Could you check a few things on this drawing? It's one solid part, dimensions in mm from its lowest x, y, z. A direction names the side the tool comes from. Give positions to 0.01 mm unless a question says otherwise; leave off trailing zeros. Order: outer loops, then holes, each group sorted by start corner. A loop starts at its lowest first (then second) coordinate and runs counter-clockwise, first axis right, second up.
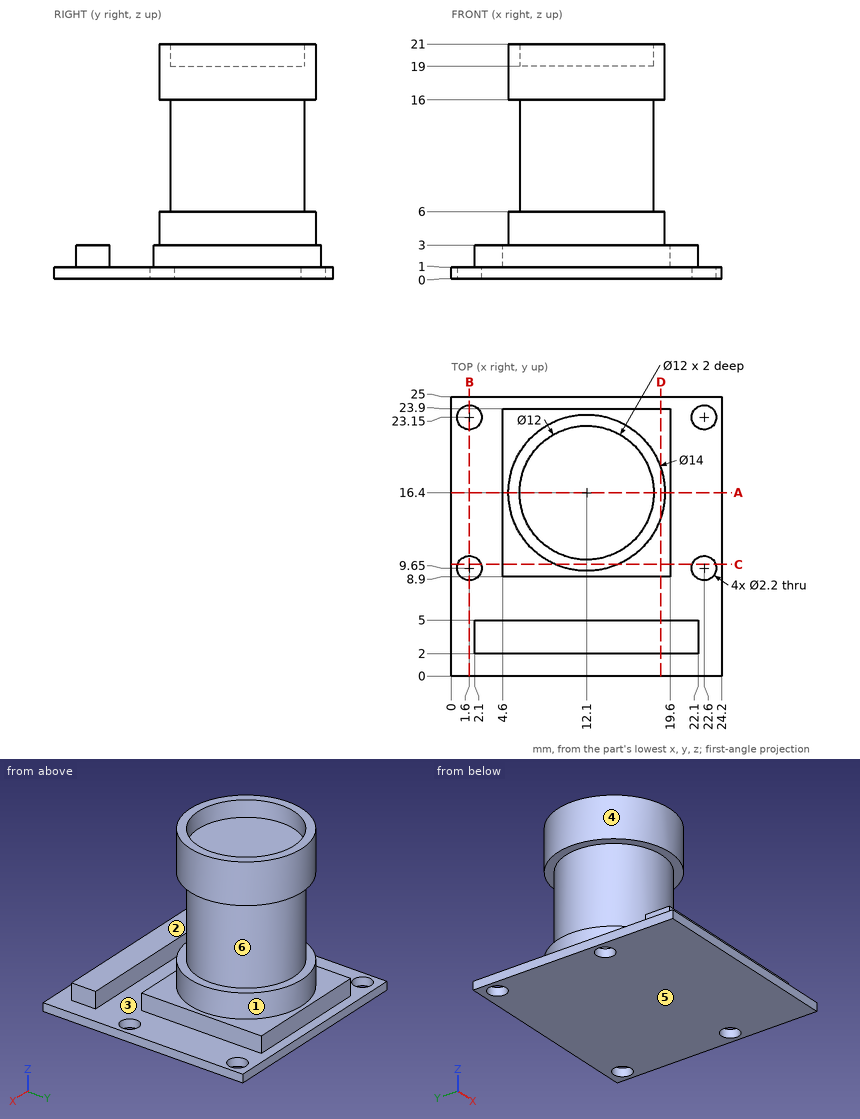
Item 1: Imagine slicing it at C-C on y = 10. List the corners of the cut face in (x, z) for me.
Findings:
outline: (0, 0) - (0.56, 0) - (0.56, 1) - (0, 1) - close; (2.64, 0) - (21.56, 0) - (21.56, 1) - (19.6, 1) - (19.6, 3) - (14.94, 3) - (14.94, 6) - (9.26, 6) - (9.26, 3) - (4.6, 3) - (4.6, 1) - (2.64, 1) - close; (9.26, 16) - (14.94, 16) - (14.94, 21) - (9.26, 21) - close; (23.64, 0) - (24.2, 0) - (24.2, 1) - (23.64, 1) - close
Item 2: Please list where these lines run through material, in increasing order: line 1 along X through (y, z) = (9.65, 0.5); line 2 along Y through (x, z) = (1.6, 0.3); line 3 along Y through (x, z) = (13.5, 2.75).
Findings:
line 1: x = 0 to 0.5, 2.7 to 21.5, 23.7 to 24.2
line 2: y = 0 to 8.55, 10.75 to 22.05, 24.25 to 25
line 3: y = 2 to 5, 8.9 to 23.9
Item 3: Imagine slicing it at D-D on x = 18.75. List the corners of the cut face in (y, z) for me.
Findings:
outline: (0, 0) - (25, 0) - (25, 1) - (23.9, 1) - (23.9, 3) - (18.59, 3) - (18.59, 6) - (14.21, 6) - (14.21, 3) - (8.9, 3) - (8.9, 1) - (5, 1) - (5, 3) - (2, 3) - (2, 1) - (0, 1) - close; (14.21, 16) - (18.59, 16) - (18.59, 21) - (14.21, 21) - close
Item 4: For the marked faces 4, 5 and 6, which set-ups out of +Z, -Z, +X, -X, +Y, -Y let a thin tool reach every point of the face, with its end or its side?
Findings:
face 4: +Z
face 5: -Z, +X, -X, +Y, -Y
face 6: none
Item 5: Imagine slicing it at A-A on y = 16.4. List the corners of the cut face in (x, z) for me, then the cut area to 3 significant figures.
Findings:
outline: (0, 0) - (24.2, 0) - (24.2, 1) - (19.6, 1) - (19.6, 3) - (19.1, 3) - (19.1, 6) - (18.1, 6) - (18.1, 16) - (19.1, 16) - (19.1, 21) - (18.1, 21) - (18.1, 19) - (6.1, 19) - (6.1, 21) - (5.1, 21) - (5.1, 16) - (6.1, 16) - (6.1, 6) - (5.1, 6) - (5.1, 3) - (4.6, 3) - (4.6, 1) - (0, 1) - close
area: 262 mm2
Item 6: For pin 1 (1 mm diameter, centred on x = 14.5, y = 5, fed in from +Z); pin 2 (2 mm diameter, centred on x = 2.5, z = 15, fed in from -Y); pin 3 (1.5 mm diameter, centred on y = 4, z = 2.5, fed in from -X); pin 4 (10 mm diameter, centred on y = 21.5, z = 10.5, fed in from +X), each with a flat end and sliding along its axis, tell me the tip position at first contact or that it passes through.
Findings:
pin 1: stops at z = 3
pin 2: passes through
pin 3: stops at x = 2.1
pin 4: stops at x = 18.46
Item 7: We'd pull the mould along Y, two halves only. Please class the marked faces 1, 2 and 3: +Y half, -Y half, draft (parallel to the pull), parting line (faces both ways), or undercut.
Findings:
face 1: parting line
face 2: draft
face 3: undercut
Item 8: Imagine slicing it at B-B on x = 1.6. List the corners of the cut face in (y, z) for me, then the cut area to 3 significant figures.
Findings:
outline: (0, 0) - (8.55, 0) - (8.55, 1) - (0, 1) - close; (10.75, 0) - (22.05, 0) - (22.05, 1) - (10.75, 1) - close; (24.25, 0) - (25, 0) - (25, 1) - (24.25, 1) - close
area: 20.6 mm2
